For this review, use the dimensioned drawing (mm, ordinates from the lowest corner) and the shaded views. A direction names the side the tool comes from. Give positions to 0.01 mm unless a question says otherwise; leave off trailing zeros. Order: outer loops, then holes, each group sorted by start corner. A loop starts at its lowest first (then second) coordinate and runs counter-clockwise, first axis right, second up. Notation, with made-up numbers: (30, -23) - (74, -23) arc R18 ccw to (74, -14) - close; hole circle Ø3 at (61.25, 8.25). An arc over 180 degrees is marked (long way). One line per item, written item: value.
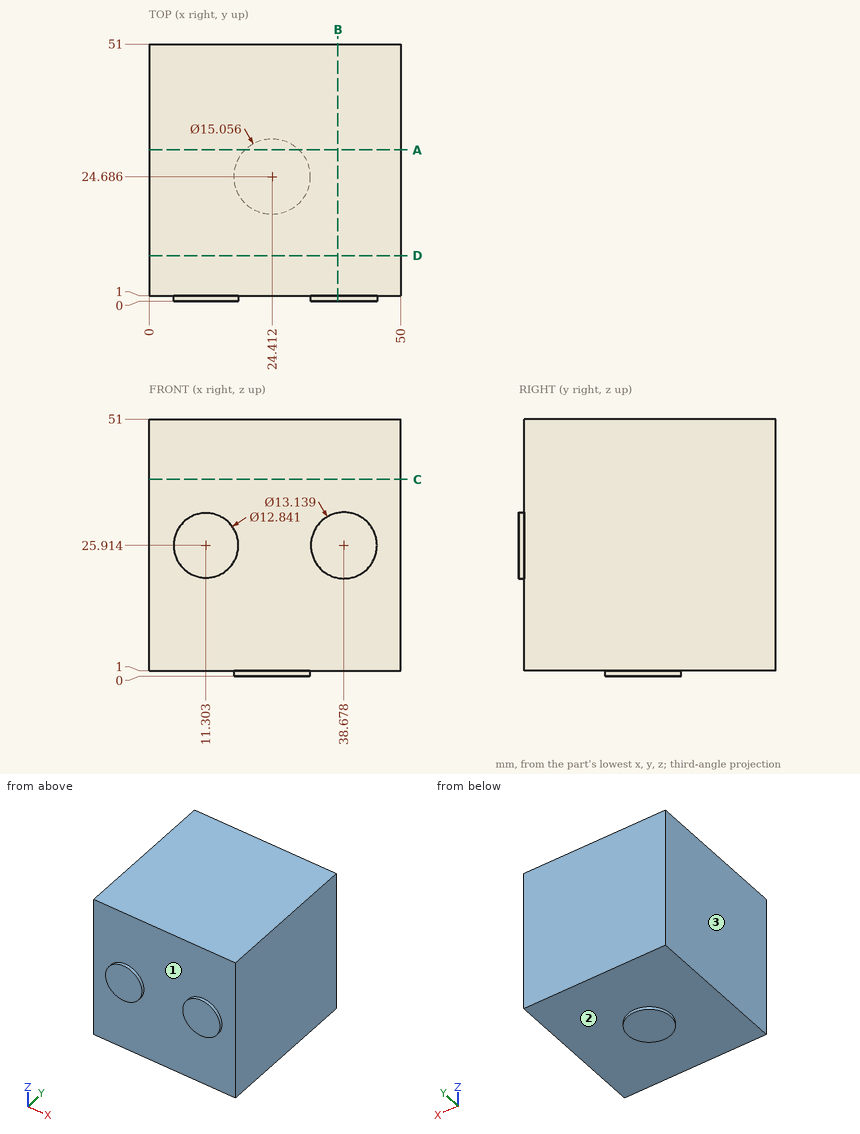
(1) Take a section at C-C (z = 39). Write out the cut boundary in (x, y).
Answers below:
outline: (0, 1) - (50, 1) - (50, 51) - (0, 51) - close
(2) Take a section at A-A (y = 30). Write out the cut boundary in (x, z) (1 decimal), then the cut area to 3 significant figures.
Answers below:
outline: (0, 1) - (19.1, 1) - (19.1, 0) - (29.7, 0) - (29.7, 1) - (50, 1) - (50, 51) - (0, 51) - close
area: 2,510 mm^2
(3) For P1, Ø2, axis at x = 39, z = 9, coming from the -Y side; P2, Ø25, axis at x = 25, z = 32, coming from the -Y side, all flat-tipped, find the tip position at first contact; note any pin that passes through.
Answers below:
P1: stops at y = 1
P2: stops at y = 0
(4) Machinability: for the marked faces 1, 2 and 3, which of the approach directions +Z, -Z, +X, -X, +Y, -Y give a long, thin tool a straight path to every point of the face, cutting with its end or side? Answer none if there is none.
Answers below:
face 1: -Y
face 2: -Z
face 3: +Z, -Z, -X, +Y, -Y
(5) Take a section at B-B (x = 37.5). Write out the cut boundary in (y, z).
Answers below:
outline: (0, 19.45) - (1, 19.45) - (1, 1) - (51, 1) - (51, 51) - (1, 51) - (1, 32.38) - (0, 32.38) - close
(6) Wall thickness on line 1 (Y direction, x = 24.5, z = 34.5): over which ranges is the line inside the solid? List them lowest first. Write a range as from..to.
Answers below:
line 1: y = 1..51
